Can you work these out from the model? Positions are in its coordinate system, mm. A direction names the side the tool comes from. Coordinates: 2 decimals unless noted, no trailing zeros. Order: outer loops, then holes, each group sorted by start corner. A loop starts at its lowest first (then second) coordinate and runs counter-clockwise, first axis right, second up. Notation, with made-up numbers: (80, -5) - (137, -5) arc R19 cw to (137, 17) - close; hole circle Ø4 at (15, 49). An arc over 180 degrees is marked (long way). Use a Markdown table: item, result. Add a question column.
(1) I want a section at D-D (y = 80). State how many separate pieces and enclosed holes the cut face has, and give its area (3 significant figures).
(2) On a 3-axis mill with a long thin cutter (end or side, diameter ignored), from which of +Z, -Z, +X, -X, +Y, -Y can I reach the whole of each face in a straight line? I mean faces 5 (the flat face through (23, 53, 31.75)), 6 (the flat face through (6.69, 39.95, -12.66)), 7 (the flat face through (-39.033, 52.55, 4.107)), 8 (the flat face through (-11.537, 52.55, 19.982)). Say none if no direction works.
(3) For pin 1 Ø10 at (y, z) = (80, -4) entering from +X; pin 2 Ø1 at (x, y) = (29, 58.5) entering from -Z; pin 3 Ø5 at (x, y) = (-3.5, 16) entering from -Z, each with a flat end and sliding along its axis, tell me the tip position at first contact or that it passes through.
(4) I want a section at C-C (x = 44.5). List the corners of the cut face in (y, z) for me, and give its area (3 significant figures).
(5) If I drill on L1, parallel to Y at x = 27, z = -12; L2, parallel to Y at x = 22.86, z = 24.5; L3, parallel to Z at x = 18.5, y = 46.5, over which ranges is the centre line in solid material (lowest first)? Write a range as [from, to].
(6) I want a section at A-A (y = 6). List the corners of the cut face in (x, z) for me, and give its area (3 significant figures).
(7) We'd pull the mould along Y, two halves only. Please class faces 1 (the flat face through (-24.88, 78.53, 11.79)), 2 (the flat face through (7.62, 40, 12)), 3 (the cylindrical face through (0.145, 59.618, -32.079)), 4 (the cylindrical face through (-5.7, 70.708, -22.025)): pulls with the +Y half, pulls with the -Y half, needs draft (parallel to the pull), parting line crosses it, or undercut.
(8) I want a section at B-B (y = 20.5). List the corners of the cut face in (x, z) for me.
```python
from build123d import *

# Parameters (mm, degrees)
SKETCH1_R           = 50.8
BOSS_EXTRUDE1_DEPTH = 25.4
SKETCH2_R           = 1.27
CUT_EXTRUDE1_DEPTH  = 12.7
BOSS_EXTRUDE2_DEPTH = 31.75
SKETCH9_R           = 6.604
CUT_EXTRUDE2_DEPTH  = 68.58
SKETCH10_R          = 1.27
CUT_EXTRUDE3_DEPTH  = 68.58
CIRPATTERN3_COUNT   = 3


with BuildPart() as part:
    # Sketch1 → Boss-Extrude1 (new body)
    with BuildSketch(Plane(origin=(0, 0, 0), x_dir=(1, 0, 0), z_dir=(0, 1, 0))):
        with Locations(Location((0, 0, 0), (0, 0, 270))):
            Circle(SKETCH1_R)
    extrude(amount=BOSS_EXTRUDE1_DEPTH)

    # Sketch2 → Cut-Extrude1 (cut)
    with BuildSketch(Plane.XZ):
        with Locations(Location((-25.4, 0, 0), (0, 0, 270))):
            Circle(SKETCH2_R)
        with Locations(Location((0, 25.4, 0), (0, 0, 270))):
            Circle(SKETCH2_R)
        with Locations(Location((25.4, 0, 0), (0, 0, 270))):
            Circle(SKETCH2_R)
        with Locations(Location((0, -25.4, 0), (0, 0, 270))):
            Circle(SKETCH2_R)
    extrude(amount=-CUT_EXTRUDE1_DEPTH, mode=Mode.SUBTRACT)

    # Sketch4 → Boss-Extrude2 (add)
    with BuildSketch(Plane.XY):
        Polygon((7.62, 25.4), (7.62, 63.5), (38.1, 93.98), (38.1, 25.4), align=None)
    boss_extrude2 = extrude(amount=BOSS_EXTRUDE2_DEPTH)

    # Sketch9 → Cut-Extrude2 (cut)
    with BuildSketch(Plane(origin=(66.802, 66.802, 0), x_dir=(0, 0, -1), z_dir=(0.7071067811865512, 0.7071067811865439, 0))):
        with Locations(Location((-15.875, 29.160757667, 0), (0, 0, 90))):
            Circle(SKETCH9_R)
    cut_extrude2 = extrude(amount=-CUT_EXTRUDE2_DEPTH, mode=Mode.SUBTRACT)

    # Sketch10 → Cut-Extrude3 (cut)
    with BuildSketch(Plane.XY.offset(31.75)):
        with Locations((22.86, 69.85)):
            Circle(SKETCH10_R)
    cut_extrude3 = extrude(amount=-CUT_EXTRUDE3_DEPTH, mode=Mode.SUBTRACT)

    # CirPattern3: Boss-Extrude2, Cut-Extrude2, Cut-Extrude3 ×3 about axis
    cirpattern3_axis = Axis((0, 0, 0), (0, 1, 0))
    add([boss_extrude2.rotate(cirpattern3_axis, i * 360 / CIRPATTERN3_COUNT) for i in range(1, CIRPATTERN3_COUNT)])
    add([cut_extrude2.rotate(cirpattern3_axis, i * 360 / CIRPATTERN3_COUNT) for i in range(1, CIRPATTERN3_COUNT)], mode=Mode.SUBTRACT)
    add([cut_extrude3.rotate(cirpattern3_axis, i * 360 / CIRPATTERN3_COUNT) for i in range(1, CIRPATTERN3_COUNT)], mode=Mode.SUBTRACT)


solid = part.part
```
Answers follow:
| question | item | result |
|---|---|---|
| 1 | separate pieces | 3 |
| 1 | enclosed holes | 0 |
| 1 | area | 1,070 mm² |
| 2 | face 5 | +Z, +X, +Y |
| 2 | face 6 | +X, +Y |
| 2 | face 7 | -Z, -X, +Y |
| 2 | face 8 | +Z, +Y |
| 3 | pin 1 | stops at x = 38.1 |
| 3 | pin 2 | stops at z = 0 |
| 3 | pin 3 | stops at z = -50.79 |
| 4 | outline | (0, -24.5) - (25.4, -24.5) - (25.4, 24.5) - (0, 24.5) - close |
| 4 | area | 1,240 mm² |
| 5 | L1 | y = [0, 25.4] |
| 5 | L2 | y = [0, 68.58], [71.12, 78.74] |
| 5 | L3 | z = [-31.46, -19.48], [0, 31.75] |
| 6 | outline | circle Ø101.6 at (0, 0); hole circle Ø2.54 at (-25.4, 0); hole circle Ø2.54 at (0, -25.4); hole circle Ø2.54 at (0, 25.4); hole circle Ø2.54 at (25.4, 0) |
| 6 | area | 8,090 mm² |
| 7 | face 1 | pulls with the +Y half |
| 7 | face 2 | needs draft |
| 7 | face 3 | undercut |
| 7 | face 4 | undercut |
| 8 | outline | circle Ø101.6 at (0, 0) |
